Read the model definition and answer for the solid it produces. Units are mm, in the model's axes. Coordinates: 2 decimals unless noted, no trailing zeros. Write each loop counter-clockwise with the first axis right and the second up, starting at its lowest first coordinate (ties: lowest second). Pieces come first, ordered by that corner, then holes. Notation, with made-up numbers: (-22, -15.5) -> (-8, -15.5) arc R12 cw to (-8, 2.5) -> close; hole circle Ø5 at (21.25, 8). An arc over 180 degrees is marked (long way). One line per item, written item: value. Start each with the question number.
1. For a pull along X with two mould halves and no side action, classify faces 1 (the flat face through (-55, 1, 34)), 2 (the flat face through (-22.61, 1.52, 19.86)) as pulls with the +X half, pulls with the -X half, needs draft (parallel to the pull), parting line crosses it, or undercut.
2. Find section C-C, the plane z = 43.5. Write down the section's boundary in (x, y) (3 decimals).
3. Consider line 1 along Z through (x, y) = (-45, 1.8); line 2 along Z through (x, y) = (-37.5, 2.45) (3 decimals); line 3 along X through (y, z) = (1.1, 65.5). Determine where each line is inside the solid, lowest interval first.
4. Find section A-A, the plane z = 107. Write down the section's boundary in (x, y) (3 decimals).
5. Find section D-D, the plane y = 2. State how many separate pieces and enclosed holes the cut face has, and give its area (3 significant figures).
6. Find section B-B, the plane x = 14.75. Write down the section's boundary in (y, z) (3 decimals).
```python
from build123d import *

# Parameters (mm, degrees)
EXTRUDE_1_DEPTH           = 3
SKETCH_2_R                = 1.525
CUT_EXTRUDE_1_DEPTH       = 4
SKETCH_5_W                = 6.5
SKETCH_5_H                = 95
CUT_EXTRUDE_4_DEPTH       = 4
FILLET_3_R                = 2
SKETCH_7_R                = 1.525
CUT_EXTRUDE_6_DEPTH       = 10
SKETCH_10_R               = 1.525
CUT_EXTRUDE_8_DEPTH       = 10
CUT_EXTRUDE_9_DEPTH       = 1
CUT_EXTRUDE_9_DEPTH_BACK  = 4
FILLET_4_R                = 1
SKETCH_15_W               = 40
SKETCH_15_H               = 20
SKETCH_15_W_2             = 30
SKETCH_15_H_2             = 15
CUT_EXTRUDE_10_DEPTH      = 1
CUT_EXTRUDE_10_DEPTH_BACK = 4
FILLET_5_R                = 1
CUT_EXTRUDE_12_DEPTH      = 1
CUT_EXTRUDE_12_DEPTH_BACK = 4
SKETCH_19_R               = 1.525
CUT_EXTRUDE_13_DEPTH      = 10
CUT_EXTRUDE_14_DEPTH      = 10
HOLE_WIZARD_1_D           = 3.05
HOLE_WIZARD_1_DEPTH       = 100
HOLE_WIZARD_1_CSINK_D     = 6.1
HOLE_WIZARD_1_CSINK_ANGLE = 90


with BuildPart() as part:
    # 草图1 → 凸台-拉伸1 (new body)
    with BuildSketch(Plane(origin=(0, 0, 0), x_dir=(1, 0, 0), z_dir=(0, 1, 0))):
        Polygon((33, -55), (33, 0), (33, 40), (-55, 40), (-55, -111), (0, -111), (0, -55), align=None)
    extrude(amount=EXTRUDE_1_DEPTH)

    # 草图2 → 切除-拉伸1 (cut, through all)
    with BuildSketch(Plane(origin=(0, 3, 0), x_dir=(1, 0, 0), z_dir=(0, 1, 0))):
        with Locations((-37.5, -107)):
            Circle(SKETCH_2_R)
        with Locations((-17.5, -107)):
            Circle(SKETCH_2_R)
        with Locations((-37.5, -75)):
            Circle(SKETCH_2_R)
        with Locations((-17.5, -75)):
            Circle(SKETCH_2_R)
        with Locations((-42, 36)):
            Circle(SKETCH_2_R)
        with Locations((-22, 36)):
            Circle(SKETCH_2_R)
        with Locations((-5.25, 36)):
            Circle(SKETCH_2_R)
        with Locations((14.75, 36)):
            Circle(SKETCH_2_R)
    extrude(amount=-CUT_EXTRUDE_1_DEPTH, mode=Mode.SUBTRACT)

    # 草图5 → 切除-拉伸4 (cut, through all)
    with BuildSketch(Plane(origin=(0, 3, 0), x_dir=(1, 0, 0), z_dir=(0, 1, 0))):
        with Locations((29.75, -7.5)):
            Rectangle(SKETCH_5_W, SKETCH_5_H)
    extrude(amount=-CUT_EXTRUDE_4_DEPTH, mode=Mode.SUBTRACT)

    # 圆角3
    fillet_3_edges = [part.edges().sort_by_distance(p)[0] for p in [
        (0, 1.5, 111),
        (-55, 1.5, 111),
        (-55, 1.5, -40),
        (0, 1.5, 55),
        (26.5, 1.5, 55),
        (26.5, 1.5, -40),
    ]]
    fillet(fillet_3_edges, radius=FILLET_3_R)

    # 草图7 → 切除-拉伸6 (cut)
    with BuildSketch(Plane.XZ):
        with Locations((-49.25, 47.5)):
            Circle(SKETCH_7_R)
        with Locations((-49.25, -32.5)):
            Circle(SKETCH_7_R)
        with Locations((20.75, -32.5)):
            Circle(SKETCH_7_R)
        with Locations((20.75, 47.5)):
            Circle(SKETCH_7_R)
    extrude(amount=-CUT_EXTRUDE_6_DEPTH, mode=Mode.SUBTRACT)

    # 草图10 → 切除-拉伸8 (cut)
    with BuildSketch(Plane.XZ):
        with Locations((-30.25, 43.5)):
            Circle(SKETCH_10_R)
        with Locations((1.75, 43.5)):
            Circle(SKETCH_10_R)
        with Locations((-30.25028, -20.4998432)):
            Circle(SKETCH_10_R)
        with Locations((1.75, -20.5)):
            Circle(SKETCH_10_R)
    extrude(amount=-CUT_EXTRUDE_8_DEPTH, mode=Mode.SUBTRACT)

    # 草图14 → 切除-拉伸9 (cut, two sides)
    with BuildSketch(Plane(origin=(0, 3, 0), x_dir=(1, 0, 0), z_dir=(0, 1, 0))) as cut_extrude_9_sk:
        Polygon((-10.25, -7.5), (7.25, 10), (7.25, -25), align=None)
        Polygon((-31.75, 14), (3.25, 14), (-14.25, -3.5), align=None)
        Polygon((-14.25, -11.5), (3.25, -29), (-31.75, -29), align=None)
        Polygon((-18.25, -7.5), (-35.75, -25), (-35.75, 10), align=None)
    extrude(amount=CUT_EXTRUDE_9_DEPTH, mode=Mode.SUBTRACT)
    extrude(cut_extrude_9_sk.sketch, amount=-CUT_EXTRUDE_9_DEPTH_BACK, mode=Mode.SUBTRACT)

    # 圆角4
    fillet_4_edges = [part.edges().sort_by_distance(p)[0] for p in [
        (3.25, 1.5, 29),
        (-31.75, 1.5, 29),
        (-14.25, 1.5, 11.5),
        (7.25, 1.5, -10),
        (7.25, 1.5, 25),
        (-10.25, 1.5, 7.5),
        (-35.75, 1.5, 25),
        (-35.75, 1.5, -10),
        (-18.25, 1.5, 7.5),
        (-14.25, 1.5, 3.5),
        (-31.75, 1.5, -14),
        (3.25, 1.5, -14),
    ]]
    fillet(fillet_4_edges, radius=FILLET_4_R)

    # 草图15 → 切除-拉伸10 (cut, two sides)
    with BuildSketch(Plane(origin=(0, 3, 0), x_dir=(1, 0, 0), z_dir=(0, 1, 0))) as cut_extrude_10_sk:
        with Locations((-27.5, -91)):
            Rectangle(SKETCH_15_W, SKETCH_15_H)
        with Locations((-27.5, -60.5)):
            Rectangle(SKETCH_15_W_2, SKETCH_15_H_2)
    extrude(amount=CUT_EXTRUDE_10_DEPTH, mode=Mode.SUBTRACT)
    extrude(cut_extrude_10_sk.sketch, amount=-CUT_EXTRUDE_10_DEPTH_BACK, mode=Mode.SUBTRACT)

    # 圆角5
    fillet_5_edges = [part.edges().sort_by_distance(p)[0] for p in [
        (-7.5, 1.5, 81),
        (-7.5, 1.5, 101),
        (-47.5, 1.5, 101),
        (-47.5, 1.5, 81),
        (-12.5, 1.5, 53),
        (-12.5, 1.5, 68),
        (-42.5, 1.5, 68),
        (-42.5, 1.5, 53),
    ]]
    fillet(fillet_5_edges, radius=FILLET_5_R)

    # 草图17 → 切除-拉伸12 (cut, two sides)
    with BuildSketch(Plane(origin=(0, 3, 0), x_dir=(1, 0, 0), z_dir=(0, 1, 0))) as cut_extrude_12_sk:
        with BuildLine():
            Line((-19.25, 31), (-9.25, 31))
            ThreePointArc((-9.25, 31), (-3.25, 25), (-9.25, 19))
            Line((-9.25, 19), (-19.25, 19))
            ThreePointArc((-19.25, 19), (-25.25, 25), (-19.25, 31))
        make_face()
        with BuildLine():
            Line((-19.25, -46), (-9.25, -46))
            ThreePointArc((-9.25, -46), (-3.25, -40), (-9.25, -34))
            Line((-9.25, -34), (-19.25, -34))
            ThreePointArc((-19.25, -34), (-25.25, -40), (-19.25, -46))
        make_face()
    extrude(amount=CUT_EXTRUDE_12_DEPTH, mode=Mode.SUBTRACT)
    extrude(cut_extrude_12_sk.sketch, amount=-CUT_EXTRUDE_12_DEPTH_BACK, mode=Mode.SUBTRACT)

    # 草图19 → 切除-拉伸13 (cut)
    with BuildSketch(Plane(origin=(0, 3, 0), x_dir=(1, 0, 0), z_dir=(0, 1, 0))):
        with Locations((-49.25, -37.5)):
            Circle(SKETCH_19_R)
        with Locations((20.75, 22.5)):
            Circle(SKETCH_19_R)
        with Locations((-49.25, 22.5)):
            Circle(SKETCH_19_R)
        with Locations((20.75, -37.5)):
            Circle(SKETCH_19_R)
    extrude(amount=-CUT_EXTRUDE_13_DEPTH, mode=Mode.SUBTRACT)

    # 草图16 → 切除-拉伸14 (cut)
    with BuildSketch(Plane(origin=(0, 3, 0), x_dir=(1, 0, 0), z_dir=(0, 1, 0))):
        with BuildLine():
            Line((-50, -27.5), (-50, 12.5))
            ThreePointArc((-50, 12.5), (-45.375, 17.125), (-40.75, 12.5))
            Line((-40.75, 12.5), (-40.75, -27.5))
            ThreePointArc((-40.75, -27.5), (-45.375, -32.125), (-50, -27.5))
        make_face()
        with BuildLine():
            Line((12.25, -27.5), (12.25, 12.5))
            ThreePointArc((12.25, 12.5), (16.875, 17.125), (21.5, 12.5))
            Line((21.5, 12.5), (21.5, -27.5))
            ThreePointArc((21.5, -27.5), (16.875, -32.125), (12.25, -27.5))
        make_face()
    extrude(amount=-CUT_EXTRUDE_14_DEPTH, mode=Mode.SUBTRACT)

    # 孔1
    with Locations(Plane(origin=(20.75, 3, 37.5), x_dir=(0, 0, 1), z_dir=(0, 1, 0))):
        with Locations((0, 0), (-60, -70), (0, -70), (-60, 0)):
            CounterSinkHole(HOLE_WIZARD_1_D / 2, HOLE_WIZARD_1_CSINK_D / 2, depth=HOLE_WIZARD_1_DEPTH, counter_sink_angle=HOLE_WIZARD_1_CSINK_ANGLE)


solid = part.part
```
Answer block:
1. face 1: pulls with the -X half
1. face 2: undercut
2. outline: (-55, 0) -> (-31.775, 0) -> (-31.775, 3) -> (-55, 3) -> close; (-28.725, 0) -> (-24.123, 0) -> (-24.123, 3) -> (-28.725, 3) -> close; (-4.377, 0) -> (0.225, 0) -> (0.225, 3) -> (-4.377, 3) -> close; (3.275, 0) -> (26.5, 0) -> (26.5, 3) -> (3.275, 3) -> close
3. line 1: z = -40 to -17.11, 32.11 to 81, 101 to 111
3. line 2: z = -40 to 53, 68 to 73.475, 76.525 to 81, 101 to 105.475, 108.525 to 111
3. line 3: x = -55 to -42.5, -12.5 to 0
4. outline: (-55, 0) -> (-39.025, 0) -> (-39.025, 3) -> (-55, 3) -> close; (-35.975, 0) -> (-19.025, 0) -> (-19.025, 3) -> (-35.975, 3) -> close; (-15.975, 0) -> (0, 0) -> (0, 3) -> (-15.975, 3) -> close
5. separate pieces: 1
5. enclosed holes: 30
5. area: 6,850 mm2
6. outline: (0, -40) -> (3, -40) -> (3, -37.525) -> (0, -37.525) -> close; (0, -34.475) -> (3, -34.475) -> (3, -16.608) -> (0, -16.608) -> close; (0, 31.608) -> (3, 31.608) -> (3, 55) -> (0, 55) -> close
